For this review, take the finished solid that the model builds, in its own axes (mm). A direction names the side the tool comes from. Coordinates: 2 decimals unless noted, no trailing zeros. Loops run counter-clockwise (first coordinate to the right, second up) from the corner with the lowest first, then second, coordinate; pieces in that order, holes last. Notation, with made-up numbers: (38.5, -21) - (73.5, -21) arc R14 cw to (73.5, -14) - close; hole circle Ø6 at (58, 15). An arc over 180 degrees is marked (long way). One line per item, written item: value. Start each with the question number.
1. Take a section at C-C, the plane z = 3. State the section outline as (x, y) points.
2. For faces 5 (the face through (26, 11.838, 14)), 6 (the face through (18, -32, 4.5)), 7 (the face through (12, 11.838, 2)), list the 3-axis set-ups (+Z, -Z, +X, -X, +Y, -Y) from which the entire face can be reached by the end or side of a thin tool; tool diameter is ignored.
3. Take a section at D-D, the plane y = 0. State the section outline as (x, z) points, and give its area (3 significant figures).
4. Insertion check: pin 1 (6 mm diameter, centred on y = 3, z = 31, fed in from -X); pin 2 (12 mm diameter, centred on x = 17.5, y = 10.5, fed in from +Z); pin 3 (5 mm diameter, centred on x = 20, y = 20, fed in from +Z); pin 4 (4 mm diameter, centred on x = 18.23, y = -29.41, fed in from +Z). Each pin has a flat end and moves straight along its axis. Give the tip position at first contact, or say it passes through.
5. The part is to be moulded in two halves that separate along Y. For faces 1 (the face through (25.827, -1.457, 35.854)), 2 (the face through (20.046, -21.736, 2.535)), 3 (the face through (26, -23.162, 14)), 4 (the face through (24, 18, 5)), say which applies: released by +Y, released by -Y, zero draft, split by the parting line, or undercut.
6. To check wall thickness, follow line 1 (Y direction, x = 13.5, z = 3); line 2 (Y direction, x = 28.5, z = 22.5); line 3 (Z direction, x = 28.5, y = -27). State the ranges of each line that lie inside material, in increasing order. Write a range as from..to.
7. Take a section at B-B, the plane y = 19. State the section outline as (x, z) points.
8. Take a section at A-A, the plane z = 27. State the section outline as (x, y) points.
```python
from build123d import *

# Parameters (mm, degrees)
EXTRUDE_2_DEPTH                = 5
SKETCH_4_W                     = 8.676470589
SKETCH_4_H                     = 35
SKETCH_4_W_2                   = 8.676470588
EXTRUDE_15_DEPTH               = 35
CUT_EXTRUDE_1_DEPTH            = 45
SKETCH_6_R                     = 14
CUT_EXTRUDE_2_DEPTH            = 45
FILLET_1_R                     = 5
SKETCH_7_R                     = 15
SKETCH_7_R_2                   = 13
EXTRUDE_16_DEPTH               = 1
SPLIT_BODIES_1_SURFACE_1_BACK  = 86
SPLIT_BODIES_1_SURFACE_1_DEPTH = 172
SPLIT_BODIES_1_SURFACE_2_BACK  = 86
SPLIT_BODIES_1_SURFACE_2_DEPTH = 172
HOLE_WIZARD_1_D                = 4.3
HOLE_WIZARD_1_DEPTH            = 5
HOLE_WIZARD_1_CBORE_D          = 10
HOLE_WIZARD_1_CBORE_DEPTH      = 0.5
HOLE_WIZARD_1_TIP              = 1.291850331


with BuildPart() as part:
    # 草图2 → 凸台-拉伸2 (new body)
    with BuildSketch(Plane.XY):
        Polygon((7.726423565, 24.338235294), (-14.773576435, 24.338235294), (-14.773576435, -35.661764706), (7.726423565, -35.661764706), (7.726423565, -23.161764706), (-6.097105846, -23.161764706), (-6.097105846, 11.838235294), (7.726423565, 11.838235294), align=None)
        Polygon((30.226423565, 24.338235294), (7.726423565, 24.338235294), (7.726423565, 11.838235294), (21.549952977, 11.838235294), (21.549952977, -23.161764706), (7.726423565, -23.161764706), (7.726423565, -35.661764706), (30.226423565, -35.661764706), align=None)
    extrude(amount=EXTRUDE_2_DEPTH)

    # 草图4 → 凸台-拉伸15 (add)
    with BuildSketch(Plane.XY.offset(5)):
        with Locations((-10.435341141, -5.661764706)):
            Rectangle(SKETCH_4_W, SKETCH_4_H)
        with Locations((25.888188271, -5.661764706)):
            Rectangle(SKETCH_4_W_2, SKETCH_4_H)
    extrude(amount=EXTRUDE_15_DEPTH)

    # 草图5 → 切除-拉伸1 (cut)
    with BuildSketch(Plane.ZY.offset(14.773576435)):
        with BuildLine():
            Line((40, -23.161764706), (40, -5.661764706))
            ThreePointArc((40, -5.661764706), (34.874368671, -18.036133377), (22.5, -23.161764706))
            Line((22.5, -23.161764706), (40, -23.161764706))
        make_face()
        with BuildLine():
            ThreePointArc((22.5, 11.838235294), (34.874368671, 6.712603965), (40, -5.661764706))
            Line((40, -5.661764706), (40, 11.838235294))
            Line((40, 11.838235294), (22.5, 11.838235294))
        make_face()
    extrude(amount=-CUT_EXTRUDE_1_DEPTH, mode=Mode.SUBTRACT)

    # 草图6 → 切除-拉伸2 (cut)
    with BuildSketch(Plane.ZY.offset(14.773576435)):
        with Locations((22.5, -5.661764706)):
            Circle(SKETCH_6_R)
    extrude(amount=-CUT_EXTRUDE_2_DEPTH, mode=Mode.SUBTRACT)

    # 圆角1
    fillet_1_edges = [part.edges().sort_by_distance(p)[0] for p in [
        (-6.097105846, 11.838235294, 2.5),
        (-6.097105846, -23.161764706, 2.5),
        (21.549952977, -23.161764706, 2.5),
        (21.549952977, 11.838235294, 2.5),
    ]]
    fillet(fillet_1_edges, radius=FILLET_1_R)

    # 草图7 → 凸台-拉伸16 (add)
    with BuildSketch(Plane(origin=(-6.097105846, 0, 0), x_dir=(0, 0, -1), z_dir=(1, 0, 0))):
        with Locations((-22.5, -5.661764706)):
            Circle(SKETCH_7_R)
        with Locations((-22.5, -5.661764706)):
            Circle(SKETCH_7_R_2, mode=Mode.SUBTRACT)
    extrude(amount=-EXTRUDE_16_DEPTH)


with BuildPart() as body_2:
    # Split Bodies 1: the piece behind the surface
    add(part.part)
    # Split Bodies 1 surface: a surface, the sketch's curves swept straight by 172 mm
    with BuildLine(Plane.XY.offset(5).offset(-SPLIT_BODIES_1_SURFACE_1_BACK), mode=Mode.PRIVATE) as split_bodies_1_surface_1_path:
        Line((7.726423565, 24.338235294), (7.726423565, -35.661764706))
    split_bodies_1_surface_1 = Shell.extrude(split_bodies_1_surface_1_path.wire(), (0 * SPLIT_BODIES_1_SURFACE_1_DEPTH, 0 * SPLIT_BODIES_1_SURFACE_1_DEPTH, 1 * SPLIT_BODIES_1_SURFACE_1_DEPTH))
    split(bisect_by=split_bodies_1_surface_1, keep=Keep.BOTTOM)


with BuildPart() as part_1:
    add(part.part)

    # Split Bodies 1: split by a surface, the side it looks to stays
    # Split Bodies 1 surface: a surface, the sketch's curves swept straight by 172 mm
    with BuildLine(Plane.XY.offset(5).offset(-SPLIT_BODIES_1_SURFACE_2_BACK), mode=Mode.PRIVATE) as split_bodies_1_surface_2_path:
        Line((7.726423565, 24.338235294), (7.726423565, -35.661764706))
    split_bodies_1_surface_2 = Shell.extrude(split_bodies_1_surface_2_path.wire(), (0 * SPLIT_BODIES_1_SURFACE_2_DEPTH, 0 * SPLIT_BODIES_1_SURFACE_2_DEPTH, 1 * SPLIT_BODIES_1_SURFACE_2_DEPTH))
    split(bisect_by=split_bodies_1_surface_2, keep=Keep.TOP)

    # 打孔尺寸(%根据六角头螺)栓 全螺纹的类型1
    with Locations(Plane(origin=(18.226423565, 18.088235294, 5), x_dir=(1, 0, 0), z_dir=(0, 0, 1))):
        with Locations((0, 0), (0, -47.5)):
            CounterBoreHole(HOLE_WIZARD_1_D / 2, HOLE_WIZARD_1_CBORE_D / 2, HOLE_WIZARD_1_CBORE_DEPTH, depth=HOLE_WIZARD_1_DEPTH)
            with Locations((0, 0, -(HOLE_WIZARD_1_DEPTH + HOLE_WIZARD_1_TIP / 2))):  # 118° drill point
                Cone(0, HOLE_WIZARD_1_D / 2, HOLE_WIZARD_1_TIP, mode=Mode.SUBTRACT)


solid = part_1.part
```
Solutions:
1. outline: (7.73, -35.66) - (30.23, -35.66) - (30.23, 24.34) - (7.73, 24.34) - (7.73, 11.84) - (16.55, 11.84) arc R5 cw to (21.55, 6.84) - (21.55, -18.16) arc R5 cw to (16.55, -23.16) - (7.73, -23.16) - close; hole circle Ø4.3 at (18.23, -29.41); hole circle Ø4.3 at (18.23, 18.09)
2. face 5: +Z, +X, -X, +Y
2. face 6: +Z
2. face 7: +Z, -Z, -X
3. outline: (21.55, 0) - (30.23, 0) - (30.23, 9.7) - (21.55, 9.7) - close; (21.55, 35.3) - (30.23, 35.3) - (30.23, 39.06) - (21.55, 39.06) - close
3. area: 117 mm2
4. pin 1: x = 21.55
4. pin 2: z = 35.48
4. pin 3: z = 5
4. pin 4: through
5. face 1: undercut
5. face 2: undercut
5. face 3: released by -Y
5. face 4: zero draft
6. line 1: -35.66..-23.16, 11.84..24.34
6. line 2: -23.16..-19.66, 8.34..11.84
6. line 3: 0..5
7. outline: (7.73, 0) - (16.28, 0) - (16.28, 4.5) - (13.31, 4.5) - (13.31, 5) - (7.73, 5) - close; (20.17, 0) - (30.23, 0) - (30.23, 5) - (23.14, 5) - (23.14, 4.5) - (20.17, 4.5) - close
8. outline: (21.55, -22.57) - (30.23, -22.57) - (30.23, -18.92) - (21.55, -18.92) - close; (21.55, 7.6) - (30.23, 7.6) - (30.23, 11.25) - (21.55, 11.25) - close
